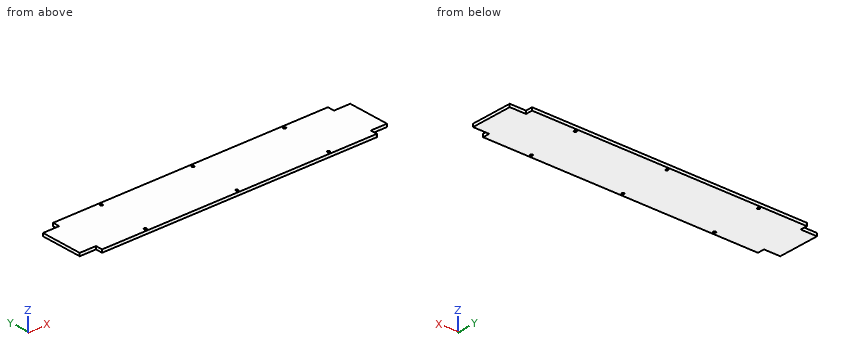
from build123d import *

# Parameters (mm, degrees)
SKETCH1_W           = 474
SKETCH1_H           = 96
BOSS_EXTRUDE1_DEPTH = 5
SKETCH2_R           = 2.1
CUT_EXTRUDE1_DEPTH  = 5
SKETCH3_W           = 28
SKETCH3_H           = 72
BOSS_EXTRUDE2_DEPTH = 5


with BuildPart() as part:
    # Sketch1 → Boss-Extrude1 (new body)
    with BuildSketch(Plane.XY):
        with Locations((237, 48)):
            Rectangle(SKETCH1_W, SKETCH1_H)
    extrude(amount=BOSS_EXTRUDE1_DEPTH)

    # Sketch2 → Cut-Extrude1 (cut)
    with BuildSketch(Plane.XY.offset(5)):
        with Locations((79, 91)):
            Circle(SKETCH2_R)
        with Locations((237, 91)):
            Circle(SKETCH2_R)
        with Locations((395, 91)):
            Circle(SKETCH2_R)
        with Locations(Location((395, 5, 0), (0, 0, 180))):
            Circle(SKETCH2_R)
        with Locations(Location((237, 5, 0), (0, 0, 180))):
            Circle(SKETCH2_R)
        with Locations(Location((79, 5, 0), (0, 0, 180))):
            Circle(SKETCH2_R)
    extrude(amount=-CUT_EXTRUDE1_DEPTH, mode=Mode.SUBTRACT)

    # Sketch3 → Boss-Extrude2 (add)
    with BuildSketch(Plane.XY.offset(5)):
        with Locations((488, 48)):
            Rectangle(SKETCH3_W, SKETCH3_H)
        with Locations((-14, 48)):
            Rectangle(SKETCH3_W, SKETCH3_H)
    extrude(amount=-BOSS_EXTRUDE2_DEPTH)


solid = part.part
Check sheet for the modelled part. Datum: model origin and axes. Units: mm. Round coordinates to 2 decimals unless told otherwise and drop trailing zeros. Order: outer loops, then holes, each group sorted by start corner. A loop starts at its lowest first (then second) coordinate and runs counter-clockwise, first axis right, second up.
(1) Scan lines: probe 1 along Y at (x, z) = (237, 2.25); probe 2 along X at (y, z) = (87, 1.25). Record each from-to range of solid material in increasing order.
(2) Go/stop test with flat-tipped pins: P1, Ø2.5, axis at y = 7.5, z = 2, coming from the +X side; P2, Ø2.5, axis at x = -12.5, z = 3.5, coming from the -Y side. Record where each tip stops, or that it passes through.
(3) Cross-section at A-A, the plane z = 3.15. Enter the section's corners in (x, y).
Check sheet entries:
1. probe 1: y = 0 to 2.9, 7.1 to 88.9, 93.1 to 96
1. probe 2: x = 0 to 474
2. P1: stops at x = 474
2. P2: stops at y = 12
3. outline: (-28, 12) - (0, 12) - (0, 0) - (474, 0) - (474, 12) - (502, 12) - (502, 84) - (474, 84) - (474, 96) - (0, 96) - (0, 84) - (-28, 84) - close; hole circle Ø4.2 at (79, 5); hole circle Ø4.2 at (79, 91); hole circle Ø4.2 at (237, 5); hole circle Ø4.2 at (237, 91); hole circle Ø4.2 at (395, 5); hole circle Ø4.2 at (395, 91)
